from build123d import *

# Parameters (mm, degrees)
F0_R      = 35
F1_DEPTH  = 8.5
F2_R      = 21.2425
F3_DEPTH  = 1
F4_R      = 21.2425
F5_DEPTH  = 6
F5_TAPER  = -30
F6_R      = 24.75
F7_DEPTH  = 1
F9_DEPTH  = 16.5
F11_DEPTH = 8.3
F12_W     = 12.0533492022
F12_H     = 52.1821774244
F12_W_2   = 10.4364354849
F12_H_2   = 52.770149804
F13_DEPTH = 8
F14_W     = 4
F14_H     = 6
F15_DEPTH = 8.5


# Not quite as in the source:
# - a pattern or mirror of a feature is missing from the dataset's text; its kind, count and spacing are read off the source's solid


with BuildPart() as f1:
    # F0 (on Front) → F1 (new body)
    with BuildSketch(Plane.XZ):
        Circle(F0_R)
    extrude(amount=F1_DEPTH)

    # F2 (on face) → F3 (join)
    with BuildSketch(Plane.XZ.offset(8.5)):
        Circle(F2_R)
    extrude(amount=F3_DEPTH)

    # F4 (on face) → F5 (join)
    with BuildSketch(Plane.XZ.offset(9.5)):
        Circle(F4_R)
    extrude(amount=F5_DEPTH, taper=F5_TAPER)

    # F6 (on face) → F7 (join)
    with BuildSketch(Plane.XZ.offset(15.5)):
        Circle(F6_R)
    extrude(amount=F7_DEPTH)

    # F8 (on face) → F9 (cut)
    with BuildSketch(Plane.XZ.offset(16.5)):
        with BuildLine():
            ThreePointArc((0, -6.9282032303), (1.4899959968, -3.6055512755), (2, 0))
            ThreePointArc((2, 0), (1.4899959968, 3.6055512755), (0, 6.9282032303))
            ThreePointArc((0, 6.9282032303), (-2, 0), (0, -6.9282032303))
        make_face()
        with BuildLine():
            ThreePointArc((0, 6.9282032303), (1.4899959968, 3.6055512755), (2, 0))
            ThreePointArc((2, 0), (1.4899959968, -3.6055512755), (0, -6.9282032303))
            ThreePointArc((0, -6.9282032303), (14.6055512755, -12.4899959968), (24, 0))
            ThreePointArc((24, 0), (14.6055512755, 12.4899959968), (0, 6.9282032303))
        make_face()
        with BuildLine():
            ThreePointArc((0, -6.9282032303), (-2, 0), (0, 6.9282032303))
            ThreePointArc((0, 6.9282032303), (-24, 0), (0, -6.9282032303))
        make_face()
    extrude(amount=-F9_DEPTH, mode=Mode.SUBTRACT)

    # F10 (on face) → F11 (cut)
    with BuildSketch(Plane.XZ.offset(16.5)):
        with BuildLine():
            ThreePointArc((0, -12.9614813968), (4.4272486205, -7.1414284285), (6, 0))
            ThreePointArc((6, 0), (4.4272486205, 7.1414284285), (0, 12.9614813968))
            ThreePointArc((0, 12.9614813968), (-6, 0), (0, -12.9614813968))
        make_face()
        with BuildLine():
            ThreePointArc((0, 12.9614813968), (4.4272486205, 7.1414284285), (6, 0))
            ThreePointArc((6, 0), (4.4272486205, -7.1414284285), (0, -12.9614813968))
            ThreePointArc((0, -12.9614813968), (18.1414284285, -15.4272486205), (28, 0))
            ThreePointArc((28, 0), (18.1414284285, 15.4272486205), (0, 12.9614813968))
        make_face()
        with BuildLine():
            ThreePointArc((0, -12.9614813968), (-6, 0), (0, 12.9614813968))
            ThreePointArc((0, 12.9614813968), (-28, 0), (0, -12.9614813968))
        make_face()
    extrude(amount=-F11_DEPTH, mode=Mode.SUBTRACT)

    # F12 (on face) → F13 (cut)
    with BuildSketch(Plane.XZ.offset(16.5)):
        with Locations((20.0266746011, 0.6560230852)):
            Rectangle(F12_W, F12_H)
        with Locations((-19.2182177424, 2.2729368025)):
            Rectangle(F12_W_2, F12_H_2)
    extrude(amount=-F13_DEPTH, mode=Mode.SUBTRACT)

    # F14 (on face) → F15 (cut)
    with BuildSketch(Plane.XZ.offset(8.5)):
        with Locations((0, 33)):
            Rectangle(F14_W, F14_H)
    f15 = extrude(amount=-F15_DEPTH, mode=Mode.SUBTRACT)

    # F15_copies: F15 across plane
    add(f15.mirror(Plane(origin=(0, 0, 0), x_dir=(-1, 0, 0), z_dir=(0, 0, -1))), mode=Mode.SUBTRACT)


solid = f1.part
CAD build for the part. Positions are in the model's coordinates, mm. A direction names the side the tool comes from. Coordinates: 2 decimals unless noted, no trailing zeros. Order: outer loops, then holes, each group sorted by start corner. A loop starts at its lowest first (then second) coordinate and runs counter-clockwise, first axis right, second up.
Item 1: Two-plate mould, pull along Y, no slides. Class faces 1 (the face through (0, -4, 30)), 2 (the face through (0, -16.5, 20)), 3 (the face through (-0.221, -11.875, -22.613)), 4 (the face through (0.221, -11.875, 22.613)): +Y half, -Y half, draft (parallel to the pull), parting line (faces both ways), or undercut.
Check sheet entries:
face 1: draft
face 2: -Y half
face 3: undercut
face 4: undercut
Item 2: Band-saw the part on A-A on y = -13. List the corners of the cut face in (x, z), plus the area to 3 significant figures.
Check sheet entries:
outline: (-14, -18.58) arc R23.26 ccw to (14, -18.58) - (14, -16.73) arc R17 cw to (0, -12.96) arc R17 cw to (-14, -16.73) - close; (-14, 16.73) arc R17 cw to (0, 12.96) arc R17 cw to (14, 16.73) - (14, 18.58) arc R23.26 ccw to (-14, 18.58) - close
area: 324 mm2
Item 3: Pin check, flat tips, straight feed: pin 1 Ø3.5 at (x, z) = (6.5, -22.5) entering from +Y; pin 2 Ø5.5 at (y, z) = (-5, 32.5) entering from -X; pin 3 Ø1.5 at (y, z) = (-5.5, 32) entering from +X; pin 4 Ø6 at (x, z) = (27, -18.5) entering from -Y. Stop position of each tip, or through.
Check sheet entries:
pin 1: stops at y = 0
pin 2: stops at x = -18.44
pin 3: stops at x = 15.76
pin 4: stops at y = -8.5
Item 4: Band-saw the part on C-C on x = -16. List the corners of the cut face in (y, z), plus the area to 3 significant figures.
Check sheet entries:
outline: (-8.5, -31.13) - (0, -31.13) - (0, -12) - (-8.2, -12) - (-8.2, -16.25) - (-8.5, -16.25) - close; (-8.5, 16.25) - (-8.2, 16.25) - (-8.2, 12) - (0, 12) - (0, 31.13) - (-8.5, 31.13) - close
area: 323 mm2
Item 5: Band-saw the part on D-D on y = -3. List the corners of the cut face in (x, z), plus the area to 3 significant figures.
Check sheet entries:
outline: (-2, -34.94) - (-2, -30) - (2, -30) - (2, -34.94) arc R35 ccw to (2, 34.94) - (2, 30) - (-2, 30) - (-2, 34.94) arc R35 ccw to start; hole (0, -6.93) arc R13 ccw (long way) to (0, 6.93) arc R13 ccw (long way) to start
area: 2,780 mm2
Item 6: Drill centre lines: L1, parallel to X at y = -2.25, z = 0; L2, parallel to Y at x = 20.5, z = -17; L3, parallel to Y at x = -26, z = -5.5. Where is each one in solid material? Low to high.
Check sheet entries:
L1: x = -35 to -24, 24 to 35
L2: y = -8.5 to 0
L3: y = -8.2 to 0
Item 7: Band-saw the part on B-B on z = -1. List the corners of the cut face in (x, y), plus the area to 3 significant figures.
Check sheet entries:
outline: (-34.99, -8.5) - (-27.97, -8.5) - (-27.97, -8.2) - (-23.96, -8.2) - (-23.96, 0) - (-34.99, 0) - close; (23.96, -8.2) - (27.97, -8.2) - (27.97, -8.5) - (34.99, -8.5) - (34.99, 0) - (23.96, 0) - close
area: 185 mm2
Item 8: 3-axis set-ups, long thin cutter, end or side, ignore diameter. For faces 5 (the face through (-0.21, -15.99, -24.75)), 6 (the face through (14, -14, -18)), 7 (the face through (-2, -4, -32)): which of +Z, -Z, +X, -X, +Y, -Y reach the whole face in a straight line?
Check sheet entries:
face 5: -Z, -Y
face 6: +Z, -Z, +X, -Y
face 7: -Z, +Y, -Y
